CAD build for the part. Positions are in the model's coordinates, mm. Give positions to 0.01 mm unless a question says otherwise; leave off trailing zeros. Order: outer loops, then holes, each group sorted by start corner. A loop starts at its lowest first (then second) coordinate and runs counter-clockwise, first axis right, second up.
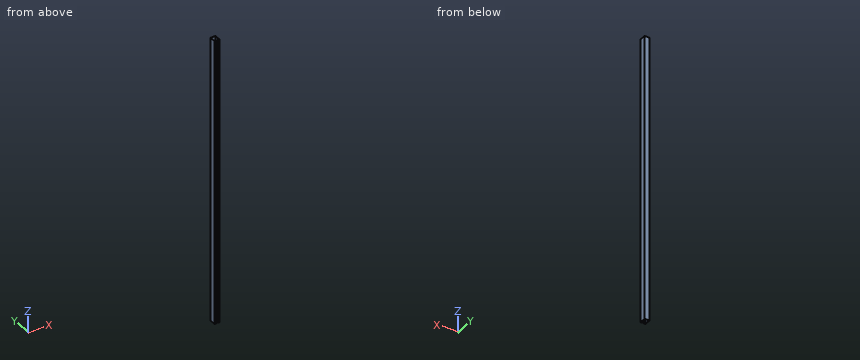
from build123d import *

# Parameters (mm, degrees)
CROQUIS1_W              = 44.45
CROQUIS1_H              = 57.15
SALIENTE_EXTRUIR1_DEPTH = 2440
CORTAR_EXTRUIR1_DEPTH   = 2440


with BuildPart() as part:
    # Croquis1 → Saliente-Extruir1 (new body)
    with BuildSketch(Plane.XY):
        with Locations((22.225, -28.575)):
            Rectangle(CROQUIS1_W, CROQUIS1_H)
    extrude(amount=SALIENTE_EXTRUIR1_DEPTH)

    # Croquis2 → Cortar-Extruir1 (cut)
    with BuildSketch(Plane.XY.offset(2440)):
        Polygon((15, -57.15), (15, -49.15), (13, -49.15), (13, -55.15), (2, -55.15), (2, -2), (42.45, -2), (42.45, -55.15), (31.45, -55.15), (31.45, -49.15), (29.45, -49.15), (29.45, -57.15), align=None)
    extrude(amount=-CORTAR_EXTRUIR1_DEPTH, mode=Mode.SUBTRACT)


solid = part.part
1. Saw through at A-A on y = -25. Give the cut face in (x, z).
2. Saw through at B-B on z = 160. Give the cut face in (x, y).
3. Wall check: line 1 (X direction, y = -51, z = 1342); line 2 (X direction, y = -35, z = 995); line 3 (Y direction, x = 31, z = 1721.5). Give the ranges that are in metal, low to high.
4. Pin check, flat tips, straight feed: P1, Ø1.5, axis at x = 24, z = 1841, coming from the -Y side; P2, Ø6, axis at x = 36.5, y = -22.5, coming from the +Z side. Stop position of each tip, or through.
Reported:
1. outline: (0, 0) - (2, 0) - (2, 2440) - (0, 2440) - close; (42.45, 0) - (44.45, 0) - (44.45, 2440) - (42.45, 2440) - close
2. outline: (0, -57.15) - (15, -57.15) - (15, -49.15) - (13, -49.15) - (13, -55.15) - (2, -55.15) - (2, -2) - (42.45, -2) - (42.45, -55.15) - (31.45, -55.15) - (31.45, -49.15) - (29.45, -49.15) - (29.45, -57.15) - (44.45, -57.15) - (44.45, 0) - (0, 0) - close
3. line 1: x = 0 to 2, 13 to 15, 29.45 to 31.45, 42.45 to 44.45
3. line 2: x = 0 to 2, 42.45 to 44.45
3. line 3: y = -57.15 to -49.15, -2 to 0
4. P1: stops at y = -2
4. P2: passes through
